Build history of the part. All positions in model axes, mm. A direction names the side the tool comes from. Give positions to 0.01 mm unless a question says otherwise; leave off trailing zeros. Loops run counter-clockwise (first coordinate to the right, second up) from the corner with the lowest first, then second, coordinate; pieces in that order, holes last. Notation, with made-up numbers: M 26,-1.75 L 68,-1.75 A33 ccw 68,26.25 Z; hole C 11.25,5 d1. An arc over 180 degrees is marked long. Answer in a Markdown table with one row per item. Add a question column.
```python
from build123d import *

# Parameters (mm, degrees)
F1_DEPTH = 10
F2_R     = 1
F3_R     = 10
F6_DEPTH = 4
F7_R     = 1


# Not quite as in the source:
# - ends of sketch curves that miss each other by under 0.0002 mm in the source are joined
# - a feature names something its author has since deleted; it is built from what else it names


with BuildPart() as f1:
    # F0 (on Top) → F1 (new body)
    with BuildSketch(Plane.XY):
        with BuildLine():
            ThreePointArc((-1.7962988307, -0.1596333839), (-12.2238763072, -14.2863823148), (-28.9155127569, -8.8376503509))
            Line((-28.9155127569, -8.8376503509), (-33.5614731624, -14.4524267481))
            Line((-33.5614731624, -14.4524267481), (-23.2513401401, -16.8024246609))
            ThreePointArc((-23.2513401401, -16.8024246609), (-11.3191539124, -17.1467252838), (-1.7954493794, -9.9498743711))
            Line((-1.7954493794, -9.9498743711), (8.2045506206, -9.9498743711))
            ThreePointArc((8.2045506206, -9.9498743711), (2.2045506206, 0), (8.2045506206, 9.9498743711))
            Line((8.2045506206, 9.9498743711), (-1.7954493794, 9.9498743711))
            ThreePointArc((-1.7954493794, 9.9498743711), (-11.3191539124, 17.1467252838), (-23.2513401401, 16.8024246609))
            Line((-23.2513401401, 16.8024246609), (-33.5614731624, 14.4524267481))
            Line((-33.5614731624, 14.4524267481), (-28.9155127569, 8.8376503509))
            ThreePointArc((-28.9155127569, 8.8376503509), (-12.3227425268, 14.3176427323), (-1.79993923, 0.3669814152))
            ThreePointArc((-1.79993923, 0.3669814152), (-1.7971307794, 0.2245866702), (-1.7956744539, 0.0821716783))
            Line((-1.7956744539, 0.0821716783), (-1.7954493794, 0.1693372455))
            Line((-1.7954493794, 0.1693372455), (-1.7954493794, 0.0497335093))
            ThreePointArc((-1.7954493794, 0.0497335093), (-1.795550035, -0.0549514122), (-1.7962988307, -0.1596333839))
        make_face()
        with BuildLine():
            Line((-1.7957105611, 0.0681883168), (-1.7962988307, -0.1596333839))
            ThreePointArc((-1.7962988307, -0.1596333839), (-1.795550035, -0.0549514122), (-1.7955318261, 0.049733236))
            Line((-1.7955318261, 0.049733236), (-1.7957105611, 0.0681883168))
        make_face()
        with BuildLine():
            Line((-1.7957105611, 0.0681883168), (-1.7954493794, 0.0497335093))
            ThreePointArc((-1.7954493794, 0.0497335093), (-1.7955943712, 0.0659524957), (-1.7956744539, 0.0821716783))
            Line((-1.7956744539, 0.0821716783), (-1.7957105611, 0.0681883168))
        make_face()
        with BuildLine():
            Line((-1.79993923, 0.3669814152), (-1.7957105611, 0.0681883168))
            Line((-1.7957105611, 0.0681883168), (-1.7956744539, 0.0821716783))
            ThreePointArc((-1.7956744539, 0.0821716783), (-1.7971307794, 0.2245866702), (-1.79993923, 0.3669814152))
        make_face()
    extrude(amount=F1_DEPTH)

    # F2
    f2_edges = [f1.edges().sort_by_distance(p)[0] for p in [
        (-33.561473, -14.452427, 5),
        (-33.561473, 14.452427, 5),
    ]]
    fillet(f2_edges, radius=F2_R)

    # F3
    f3_edges = [f1.edges().sort_by_distance(p)[0] for p in [
        (-1.795449, 9.949874, 5),
        (-1.795449, -9.949874, 5),
        (-23.25134, 16.802425, 5),
        (-23.25134, -16.802425, 5),
    ]]
    fillet(f3_edges, radius=F3_R)

    # F5 (on offset) → F6 (cut)
    with BuildSketch(Plane.XY.offset(7)):
        with BuildLine():
            ThreePointArc((11.5250723848, -12.6931975947), (0.3398769597, -1.8546317787), (7.9403583125, 11.740065307))
            Line((7.9403583125, 11.740065307), (3.2065206071, 11.740065307))
            ThreePointArc((3.2065206071, 11.740065307), (-2.2747136402, -0.7956794231), (4.4808682127, -12.6931975947))
            Line((4.4808682127, -12.6931975947), (11.5250723848, -12.6931975947))
        make_face()
    extrude(amount=-F6_DEPTH, mode=Mode.SUBTRACT)

    # F7
    f7_edges = [f1.edges().sort_by_distance(p)[0] for p in [
        (8.204551, 9.949874, 5),
        (8.204551, -9.949874, 5),
    ]]
    fillet(f7_edges, radius=F7_R)


solid = f1.part
```
(1) Slice it at B-B, the plane x = -13. Give the cut face in (y, z).
(2) Slice it at A-A, the plane z = 6.5. Give the cut face in (x, y).
(3) Pin check, flat tips, straight feed: pin 1 (5 mm diameter, centred on x = -27, z = 5, fed in from +Y); pin 2 (4 mm diameter, centred on x = -25, z = 9, fed in from +Y); pin 3 (1 mm diameter, centred on y = 8, z = 7, fed in from +X). Stop position of each tip, or through.
(4) Pull direction X, two halves, no side cores. Call faces 1 (the cylindrical face through (-12.737, 17.536, 4.93)), 2 (the cylindrical face through (-23.31, 16.806, 5.07)), 3 (the cylindrical face through (-0.806, -6.579, 5.028)): +X half, -X half, draft (parallel to the pull), parting line (faces both ways), or undercut.
(5) Tool access for faces 4 (the flat face through (0, 1, 3)), 5 (the flat face through (-30.746, 11.05, 4.93)), 6 (the flat face through (4, -9.95, 2.7)), 7 (the cylindrical face through (-12.6, 14.4, 4.9)), 8 (the flat face through (4, 9.95, 2.7)): list every direction of +Z, -Z, +X, -X, +Y, -Y with a clear straight run to the whole face (end or side of a thin tool).
(6) Slice it at D-D, the plane y = 5.5. Give the cut face in (x, z).
(7) Wall check: line 1 (Y direction, x = -13.5, z = 5.25); line 2 (Y direction, x = -11, z = 6); line 3 (X direction, y = -12.5, z = 1.5). Give the ranges that are in metal, low to high.
Solution:
| question | item | result |
|---|---|---|
| 1 | outline | M -17.6,0 L -14.51,0 L -14.51,10 L -17.6,10 Z; M 14.51,0 L 17.6,0 L 17.6,10 L 14.51,10 Z |
| 2 | outline | M -32.53,-13.2 A1 ccw -31.98,-14.81 L -23.87,-16.66 A10 cw -22.77,-16.98 A18 ccw -4.17,-12.82 A10 cw 1.47,-10.05 A15.28 cw -2.05,-2.74 A15 cw -28.92,-8.84 Z; M -32.53,13.2 L -28.92,8.84 A15 cw -2.05,2.74 A15.28 cw 1.47,10.05 A10 cw -4.17,12.82 A18 ccw -22.77,16.98 A10 cw -23.87,16.66 L -31.98,14.81 A1 ccw Z; M 4.97,-9.95 L 5.09,-9.95 A1 ccw 5.77,-8.22 A11.25 cw 5.77,8.22 A1 ccw 5.09,9.95 L 4.97,9.95 A12.78 ccw Z |
| 3 | pin 1 | y = 16.52 |
| 3 | pin 2 | y = 16.9 |
| 3 | pin 3 | x = 5.98 |
| 4 | face 1 | parting line |
| 4 | face 2 | -X half |
| 4 | face 3 | undercut |
| 5 | face 4 | none |
| 5 | face 5 | +Z, -Z, -X |
| 5 | face 6 | +Z, -Z, +X, -Y |
| 5 | face 7 | +Z, -Z |
| 5 | face 8 | +Z, -Z, +X, +Y |
| 6 | outline | M -2.84,0 L 3.64,0 L 3.64,10 L -2.84,10 Z; hole M -1.27,3 L 1.45,3 L 1.45,7 L -1.27,7 Z |
| 7 | line 1 | -17.7 to -14.63, 14.63 to 17.7 |
| 7 | line 2 | -17.04 to -13.84, 13.84 to 17.04 |
| 7 | line 3 | -31.95 to -25.09, -8.5 to -3.82 |
